The model under review builds one solid part; all positions refer to its coordinate system, in mm. A direction names the side the tool comes from. Coordinates: 2 decimals unless noted, no trailing zeros. Write each loop counter-clockwise with the first axis right and the second up, starting at its lowest first coordinate (ties: lowest second). Pieces come first, ordered by that corner, then holes.
Autodesk Inventor part; units mm, degrees
ref_plane "YZ Plane" through (0, 0, 0) normal (1, 0, 0) x (0, 1, 0)
ref_plane "XZ Plane" through (0, 0, 0) normal (0, 1, 0) x (-1, 0, 0)
ref_plane "XY Plane" through (0, 0, 0) normal (0, 0, 1) x (1, 0, 0)
sketch "Sketch1" plane through (0, 0, 0) normal (0, 0, 1) x (1, 0, 0)
  line L0 (21, -21) -> (-21, -21)
  line L1 (-21, -21) -> (-21, 21)
  line L2 (-21, 21) -> (21, 21)
  line L3 (21, 21) -> (21, -21)
  line L4 (21, -21) -> (-21, 21) construction
  line L5 (-21, -21) -> (21, 21) construction
  point P0 (0, 0)
  dimension "d0" = 42
extrude "Extrusion1" add sketch "Sketch1" along normal blind 25
sketch "Sketch2" plane through (0, 0, 25) normal (0, 0, 1) x (1, 0, 0)
  point P0 (0, 0)
  point P1 (-15.5, 15.5)
  point P2 (-15.5, -15.5)
  point P3 (15.5, -15.5)
  point P4 (15.5, 15.5)
  dimension "d3" = 31
  dimension "d4" = 31
  dimension "d5" = 15.5
  dimension "d6" = 15.5
hole "Hole1" at (-15.5, 15.5, 25) at (-15.5, -15.5, 25) at (15.5, -15.5, 25) at (15.5, 15.5, 25) direction (0, 0, -1) diameter 3 depth 8 tip angle 118
chamfer "Chamfer1" distance 3.5 angle 45 4 edges at (21, 21, 12.5) (21, -21, 12.5) (-21, 21, 12.5) (-21, -21, 12.5)
sketch "Sketch3" plane through (0, 0, 25) normal (0, 0, 1) x (1, 0, 0)
  circle A0 centre (0, 0) radius 11
  dimension "d17" = 22
extrude "Extrusion2" add sketch "Sketch3" along normal blind 2
sketch "Sketch4" plane through (0, 0, 27) normal (0, 0, 1) x (1, 0, 0)
  circle A0 centre (0, 0) radius 11
  circle A1 centre (0, 0) radius 2.5
  dimension "d20" = 5
extrude "Extrusion3" add sketch "Sketch4" along normal blind 25 contours A1
properties part number "Extruder Motor" material "Steel, Alloy"
Item 1: Machinability: for faces 5 (the face through (0, 21, 12)), 6 (the face through (-10, 10, 25)), which of the approach directions +Z, -Z, +X, -X, +Y, -Y give a long, thin tool a straight path to every point of the face, cutting with its end or side? Answer none if there is none.
Solved:
face 5: +Z, -Z, +X, -X, +Y
face 6: +Z
Item 2: Take a section at B-B, the plane y = 0. Write out the cut boundary in (x, z), plus the area to 3 significant figures.
Solved:
outline: (-21, 0) - (21, 0) - (21, 25) - (11, 25) - (11, 27) - (2.5, 27) - (2.5, 52) - (-2.5, 52) - (-2.5, 27) - (-11, 27) - (-11, 25) - (-21, 25) - close
area: 1,220 mm2
Item 3: For pin 1 (1 mm diameter, centred on x = -7, y = 2, fed in from +Z); pin 2 (3.5 mm diameter, centred on x = -15.5, y = -15.5, fed in from +Z); pin 3 (12 mm diameter, centred on y = -4.5, z = 33.5, fed in from +X), all flat-tipped, find the tip position at first contact; note any pin that passes through.
Solved:
pin 1: stops at z = 27
pin 2: stops at z = 25
pin 3: stops at x = 2.5
Item 4: Mouldability with a two-part tool opening along Y and no side actions: class faces 1 (the face through (-19.2, 19.3, 12.3)), 2 (the face through (21, 0, 12)), 3 (the face through (-15.57, 17, 20.94)), 4 (the face through (15.43, -14, 20.94)) as pulls with the +Y half, pulls with the -Y half, needs draft (parallel to the pull), parting line crosses it, or undercut.
Solved:
face 1: pulls with the +Y half
face 2: needs draft
face 3: undercut
face 4: undercut
Item 5: Take a section at D-D, the plane z = 39. Write out the cut boundary in (x, y), plus the area to 3 significant figures.
Solved:
outline: circle Ø5 at (0, 0)
area: 19.6 mm2
Item 6: To check wall thickness, follow line 1 along Y through (x, z) = (15.5, 21.75); line 2 along Y through (x, z) = (15, 23). State the ranges of each line that lie inside material, in increasing order.
Solved:
line 1: y = -21 to -17, -14 to 14, 17 to 21
line 2: y = -21 to -16.91, -14.09 to 14.09, 16.91 to 21
Item 7: Take a section at A-A, the plane z = 23. Write out the cut boundary in (x, y).
Solved:
outline: (-21, -17.5) - (-17.5, -21) - (17.5, -21) - (21, -17.5) - (21, 17.5) - (17.5, 21) - (-17.5, 21) - (-21, 17.5) - close; hole circle Ø3 at (-15.5, -15.5); hole circle Ø3 at (-15.5, 15.5); hole circle Ø3 at (15.5, -15.5); hole circle Ø3 at (15.5, 15.5)
Item 8: Take a section at C-C, the plane x = -10. Write out the cut boundary in (y, z), plus the area to 3 significant figures.
Solved:
outline: (-21, 0) - (21, 0) - (21, 25) - (4.58, 25) - (4.58, 27) - (-4.58, 27) - (-4.58, 25) - (-21, 25) - close
area: 1,070 mm2
